Design review of the part built by this model. Coordinates are the model's own, in mm. Coordinates: 2 decimals unless noted, no trailing zeros. Loops run counter-clockwise (first coordinate to the right, second up) from the corner with the lowest first, then second, coordinate; pieces in that order, holes last. Notation, with made-up numbers: (-11, -3) -> (-2, -3) arc R20 cw to (-2, 33) -> close; hole circle Ø2 at (-5.5, 35.5). An arc over 180 degrees is marked (long way). Use one line per item in the form item = value. Start each with the question number.
1. Consider section A-A (y = 0). State the section outline as (x, z) points.
2. For pin 1 (12 mm diameter, centred on x = -1, y = 4.5, fed in from -Z), flat-tipped, find the tip position at first contact; note if it passes through.
3. The part is to be moulded in two halves that separate along Y. For faces 1 (the face through (1.73, 7.81, 4.93)), 2 (the face through (0, 10, 5)), 3 (the face through (-3, 8, 0)), say which applies: released by +Y, released by -Y, zero draft, split by the parting line, or undercut.
4. Wall thickness on line 1 (Y direction, x = 0, z = 7); line 2 (X direction, y = -1, z = 2); line 3 (X direction, y = -4.25, z = 5.75): over which ranges is each line inside the solid? List them lowest first. Write a range as from..to.
5. Consider section C-C (z = 7). State the section outline as (x, y) points.
from build123d import *

# Parameters (mm, degrees)
CUT_EXTRUDE1_DEPTH      = 18.320508249
CUT_EXTRUDE1_DEPTH_BACK = 18.320508249
SKETCH3_R               = 8


with BuildPart() as part:
    # Sketch1 → Loft1 section 0
    with BuildSketch(Plane.XY):
        with BuildLine():
            Line((10, 10), (-10, 10))
            Line((-10, 10), (-10, -10))
            Line((-10, -10), (10, -10))
            Line((10, -10), (10, 10))
        make_face()
    # Sketch2 → Loft1 section 1
    with BuildSketch(Plane.XY.offset(10)):
        with BuildLine():
            Line((10, 10), (-10, 10))
            Line((-10, 10), (-10, -10))
            Line((-10, -10), (10, -10))
            Line((10, -10), (10, 10))
        make_face()
    loft()

    # Sketch3 → Cut-Extrude1 (cut, two sides: drawn at the far end of the back side and taken through both)
    with BuildSketch(Plane.XY.offset(-CUT_EXTRUDE1_DEPTH_BACK)):
        with Locations(Location((0, 0, 0), (0, 0, 180))):
            Circle(SKETCH3_R)
    extrude(amount=CUT_EXTRUDE1_DEPTH + CUT_EXTRUDE1_DEPTH_BACK, mode=Mode.SUBTRACT)


solid = part.part
Geometry check:
q1.outline = (-10, 0) -> (-8, 0) -> (-8, 10) -> (-10, 10) -> close; (8, 0) -> (10, 0) -> (10, 10) -> (8, 10) -> close
q2.pin_1 = 0
q3.face_1 = undercut
q3.face_2 = released by +Y
q3.face_3 = zero draft
q4.line_1 = -10..-8, 8..10
q4.line_2 = -10..-7.94, 7.94..10
q4.line_3 = -10..-6.78, 6.78..10
q5.outline = (-10, -10) -> (10, -10) -> (10, 10) -> (-10, 10) -> close; hole circle Ø16 at (0, 0)
